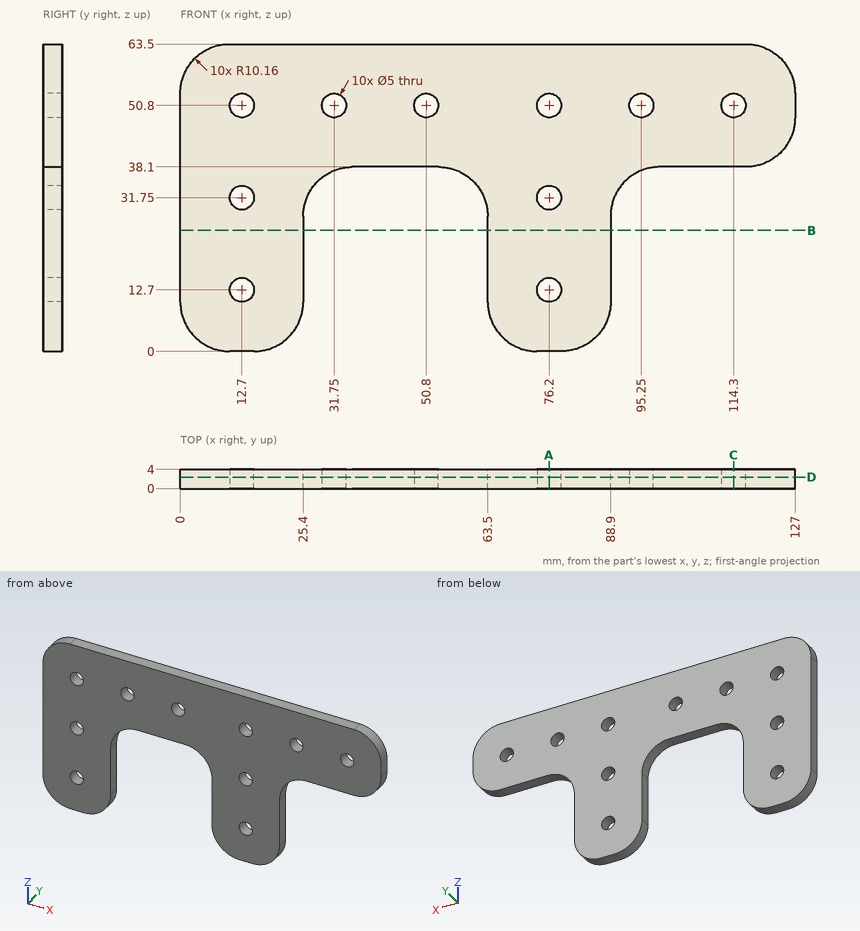
Could you check a few things on this drawing? It's one solid part, dimensions in mm from its lowest x, y, z. Round coordinates to 2 decimals unless told otherwise and drop trailing zeros. Order: outer loops, then holes, each group sorted by start corner. A loop starts at its lowest first (then second) coordinate and runs counter-clockwise, first axis right, second up. Notation, with made-up numbers: M 77,2 L 111,2 A20 ccw 111,25 Z; hole C 45,-12 d10. An arc over 180 degrees is marked long. Return JSON: item names as keys, results as strings. Group by question number.
1. If we section it at C-C on x = 114.3: List the corners of the cut face in (y, z) for me, then the cut area to 3 significant figures.
2. I'm going to push a flat-ended pin straight in: pin 1 Ø2 at (y, z) = (1.5, 18) entering from +X. Where does the tip first touch, or does it pass through?
3. If we section it at D-D on y = 2.4: State how many separate pieces and enclosed holes the cut face has, then the cut area to 3 significant figures.
4. Please list where these lines run through material, in increasing order: probe 1 along Z at (x, y) = (12.7, 1.8); probe 2 along X at (y, z) = (1.85, 12.7); probe 3 along X at (y, z) = (0.55, 20.5).
5. If we section it at A-A on x = 76.2: List the corners of the cut face in (y, z) for me, then the cut area to 3 significant figures.
6. If we section it at B-B on z = 25: List the corners of the cut face in (x, y) for me.
Reply:
{
 "1": {"outline": "M 0,38.1 L 4,38.1 L 4,48.3 L 0,48.3 Z; M 0,53.3 L 4,53.3 L 4,63.5 L 0,63.5 Z", "area": "81.6 mm^2"},
 "2": {"pin 1": "x = 88.9"},
 "3": {"separate pieces": "1", "enclosed holes": "10", "area": "4,880 mm^2"},
 "4": {"probe 1": "0 to 10.2, 15.2 to 29.25, 34.25 to 48.3, 53.3 to 63.5", "probe 2": "0 to 10.2, 15.2 to 25.4, 63.5 to 73.7, 78.7 to 88.9", "probe 3": "0 to 25.4, 63.5 to 88.9"},
 "5": {"outline": "M 0,0 L 4,0 L 4,10.2 L 0,10.2 Z; M 0,15.2 L 4,15.2 L 4,29.25 L 0,29.25 Z; M 0,34.25 L 4,34.25 L 4,48.3 L 0,48.3 Z; M 0,53.3 L 4,53.3 L 4,63.5 L 0,63.5 Z", "area": "194 mm^2"},
 "6": {"outline": "M 0,0 L 25.4,0 L 25.4,4 L 0,4 Z; M 63.5,0 L 88.9,0 L 88.9,4 L 63.5,4 Z"}
}
